from build123d import *

# Parameters (mm, degrees)
IZIM1_W                     = 30
IZIM1_H                     = 30
Y_KSEKLIK_EKSTR_ZYON1_DEPTH = 36
IZIM3_W                     = 18
IZIM3_H                     = 18
KES_EKSTR_ZYON2_DEPTH       = 55.968631837
IZIM5_R                     = 5
KES_EKSTR_ZYON3_DEPTH       = 55.968631837
IZIM6_W                     = 9
IZIM6_H                     = 30
Y_KSEKLIK_EKSTR_ZYON2_DEPTH = 34
RADYUS1_R                   = 15
IZIM7_R                     = 7.5
KES_EKSTR_ZYON4_DEPTH       = 80


with BuildPart() as part:
    # Çizim1 → Yükseklik-Ekstrüzyon1 (new body)
    with BuildSketch(Plane(origin=(0, 0, 0), x_dir=(1, 0, 0), z_dir=(0, 1, 0))):
        with Locations((13.732394366, 15)):
            Rectangle(IZIM1_W, IZIM1_H)
    extrude(amount=Y_KSEKLIK_EKSTR_ZYON1_DEPTH)

    # Çizim3 → Kes-Ekstrüzyon2 (cut, through all)
    with BuildSketch(Plane.XY):
        with Locations((19.732394366, 18)):
            Rectangle(IZIM3_W, IZIM3_H)
    extrude(amount=-KES_EKSTR_ZYON2_DEPTH, mode=Mode.SUBTRACT)

    # Çizim5 → Kes-Ekstrüzyon3 (cut, through all)
    with BuildSketch(Plane(origin=(0, 36, 0), x_dir=(1, 0, 0), z_dir=(0, 1, 0))):
        with Locations((-1.267605634, 15)):
            Circle(IZIM5_R)
    extrude(amount=-KES_EKSTR_ZYON3_DEPTH, mode=Mode.SUBTRACT)

    # Çizim6 → Yükseklik-Ekstrüzyon2 (add)
    with BuildSketch(Plane(origin=(0, 36, 0), x_dir=(1, 0, 0), z_dir=(0, 1, 0))):
        with Locations((24.232394366, 15)):
            Rectangle(IZIM6_W, IZIM6_H)
    extrude(amount=Y_KSEKLIK_EKSTR_ZYON2_DEPTH)

    # Radyus1
    radyus1_edges = [part.edges().sort_by_distance(p)[0] for p in [
        (24.232394366, 70, 0),
        (24.232394366, 70, -30),
    ]]
    fillet(radyus1_edges, radius=RADYUS1_R - 0.0001)  # a hair under: the kernel refuses the full size

    # Çizim7 → Kes-Ekstrüzyon4 (cut, through all)
    with BuildSketch(Plane.ZY.offset(-19.732394366)):
        with Locations((-15, 57.087838251)):
            Circle(IZIM7_R)
    extrude(amount=-KES_EKSTR_ZYON4_DEPTH, mode=Mode.SUBTRACT)


solid = part.part
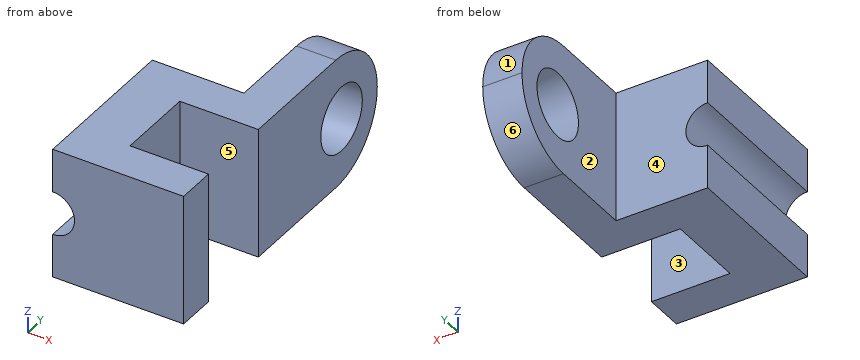
For this review, take the finished solid that the model builds, in its own axes (mm). Face numbers are marked on the shaded views. A direction names the side the tool comes from. Give positions to 0.01 mm unless a question says otherwise; leave off trailing zeros. Loops run counter-clockwise (first coordinate to the right, second up) from the corner with the lowest first, then second, coordinate; pieces in that order, holes last.
Item 1: Take a section at D-D, the plane z = -2.5. State the section outline as (x, y) points, and give its area (3 significant figures).
Item 2: Take a section at C-C, the plane y = 21.5. State the section outline as (x, z) points, and give its area (3 significant figures).
Item 3: Draft analysis for pull direction Y (two halves, no side actions). For the marked faces 1, 2 and 3, state which applies: +Y half, -Y half, draft (parallel to the pull), parting line (faces both ways), or undercut.
Item 4: Take a section at B-B, the plane x = 14. State the section outline as (y, z) points, and give its area (3 significant figures).
Item 5: Take a section at A-A, the plane x = 21. Give the number of separate pieces and of enclosed holes in the cut face, and give its area (3 significant figures).
Item 6: Insertion check: pin 1 (5 mm diameter, centred on x = 2.5, z = -5.5, fed in from +Y); pin 2 (6 mm diameter, centred on y = 21, z = -19, fed in from +X); pin 3 (9 mm diameter, centred on y = 54, z = -22, fed in from -X). Each pin has a flat end and moves straight along its axis. Give the tip position at first contact, or say it passes through.
Item 7: For line 1 along Y through (x, z) = (25, -15); line 2 along Y through (x, z) = (16, -8.5); line 3 along Y through (x, z) = (0, -26.5), list the stretches that pass through material, from the lowest coordinate up.
Item 8: Tool access review of the marked faces 4, 5 and 6: name each direction out of +Z, -Z, +X, -X, +Y, -Y from which nothing blocks a thin tool from reaching the whole face with its end or side.
Calculated:
1. outline: (-1.27, 0) - (28.73, 0) - (28.73, 9) - (10.73, 9) - (10.73, 27) - (28.73, 27) - (28.73, 63.29) - (19.73, 63.29) - (19.73, 36) - (-1.27, 36) - close
1. area: 1,000 mm2
2. outline: (-1.27, -30) - (10.73, -30) - (10.73, 0) - (-1.27, 0) - (-1.27, -10) arc R5 cw to (-1.27, -20) - close
2. area: 321 mm2
3. face 1: +Y half
3. face 2: draft
3. face 3: undercut
4. outline: (0, -30) - (9, -30) - (9, 0) - (0, 0) - close; (27, -30) - (36, -30) - (36, 0) - (27, 0) - close
4. area: 540 mm2
5. separate pieces: 2
5. enclosed holes: 1
5. area: 1,290 mm2
6. pin 1: stops at y = 36
6. pin 2: stops at x = 10.73
6. pin 3: stops at x = 19.73
7. line 1: y = 0 to 9, 27 to 49.59, 64.59 to 70
7. line 2: y = 0 to 9, 27 to 36
7. line 3: y = 0 to 36
8. face 4: +Z, -Z, -X, +Y
8. face 5: +Z, -Z, +X
8. face 6: -Z, +X, -X, +Y
